Print and shaded views of the part. All mm, measured from the part's lowest x, y and z. A direction names the side the tool comes from. Give positions to 0.01 mm unless a question says otherwise; leave off trailing zeros. Order: outer loops, then holes, each group sorted by start corner. A loop starts at its lowest first (then second) coordinate and runs counter-clockwise, first axis right, second up. Notation, with made-up numbers: (81.5, -10.5) -> (132.5, -10.5) arc R20 ccw to (132.5, 21.5) -> close; hole circle Ø2 at (-35.75, 7). An arc over 180 degrees is marked (long way). One line per question, with ' | ' between items. Start each with the question number.
(1) Which spindle directions (+Z, -Z, +X, -X, +Y, -Y) get a long thin tool onto all of the face, cutting with end or side? Do the marked faces 1 and 2. Say none if no direction does.
(2) Cut at D-D (y = 2.75). Give the cut face in (x, z).
(3) Pull direction X, two halves, no side cores. Call the marked faces 3, 4 and 5: +X half, -X half, draft (parallel to the pull), parting line (faces both ways), or undercut.
(4) Cut at B-B (x = 6.5). Give the cut face in (y, z).
(5) Drill centre lines: L1, parallel to Y at x = 10.25, z = 8.5; L2, parallel to Y at x = 10.5, z = 2.5; L3, parallel to X at y = 6.5, z = 10.5 (1 decimal). Where is each one in solid material? Low to high. Write a range as from..to.
(6) Cut at A-A (z = 9.25). Give the cut face in (x, y) (1 decimal), then the cut area to 3 significant figures.
(7) Pin check, flat tips, straight feed: pin 1 Ø6 at (x, z) = (4, 9.5) entering from -Y; pin 2 Ø2 at (y, z) = (13.5, 3.5) entering from +X; pin 3 Ø4 at (y, z) = (12, 2) entering from -X. Stop position of each tip, or through.
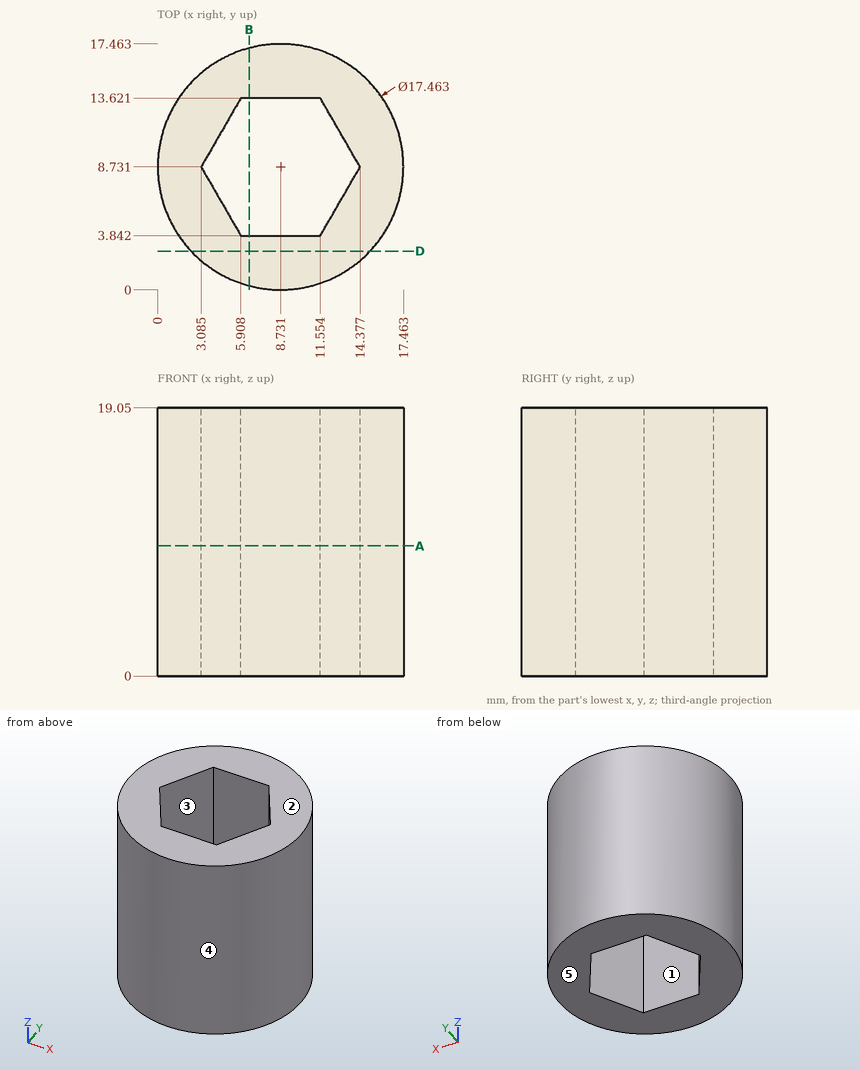
Result set:
1) face 1: +Z, -Z | face 2: +Z, +X, -X, +Y, -Y
2) outline: (2.37, 0) -> (15.09, 0) -> (15.09, 19.05) -> (2.37, 19.05) -> close
3) face 3: undercut | face 4: parting line | face 5: draft
4) outline: (0.29, 0) -> (3.84, 0) -> (3.84, 19.05) -> (0.29, 19.05) -> close; (13.62, 0) -> (17.17, 0) -> (17.17, 19.05) -> (13.62, 19.05) -> close
5) L1: y = 0.13..3.84, 13.62..17.33 | L2: y = 0.18..3.84, 13.62..17.28 | L3: x = 0.3..4.4, 13.1..17.2
6) outline: circle Ø17.5 at (8.7, 8.7); hole (3.1, 8.7) -> (5.9, 3.8) -> (11.6, 3.8) -> (14.4, 8.7) -> (11.6, 13.6) -> (5.9, 13.6) -> close | area: 157 mm2
7) pin 1: stops at y = 0.17 | pin 2: stops at x = 16.61 | pin 3: stops at x = 0.09
